```python
from build123d import *

# Parameters (mm, degrees)
F1_DEPTH   = 25.4
F2_DEPTH   = 6.35
F4_DEPTH   = 25.4
F5_DEPTH   = 25.4
F2_FACE2_W = 0.635
F2_FACE2_H = 6.35
F2_FACE3_W = 10.16
F2_FACE3_H = 6.35
F7_DEPTH   = 25.4
F9_DEPTH   = 25.4


with BuildPart() as f1:
    # F0 (on Top) → F1 (new body)
    with BuildSketch(Plane.XY):
        with BuildLine():
            ThreePointArc((1.2208780752, -0.3497952621), (1.2576595635, -0.1766137657), (1.27, 0))
            ThreePointArc((1.27, 0), (1.0317462976, 0.7405400579), (0.4063786184, 1.2032275007))
            ThreePointArc((0.4063786184, 1.2032275007), (0.0082488661, 1.2699732108), (-0.3907143254, 1.2084048642))
            ThreePointArc((-0.3907143254, 1.2084048642), (-1.1197739724, 0.5991713033), (-1.2221285, -0.3454011139))
            ThreePointArc((-1.2221285, -0.3454011139), (-1.0969705534, -0.6399653154), (-0.9021458423, -0.8938863906))
            ThreePointArc((-0.9021458423, -0.8938863906), (-0.0022842997, -1.2699979457), (0.8989244127, -0.897125911))
            ThreePointArc((0.8989244127, -0.897125911), (1.0946612978, -0.643907325), (1.2208780752, -0.3497952621))
        make_face()
    extrude(amount=F1_DEPTH)

    # F0 (on Top) → F2 (join)
    with BuildSketch(Plane.XY):
        with BuildLine():
            ThreePointArc((-0.9021458423, -0.8938863906), (-1.0969705534, -0.6399653154), (-1.2221285, -0.3454011139))
            Line((-1.2221285, -0.3454011139), (-10.0618945001, -5.3538077531))
            Line((-10.0618945001, -5.3538077531), (-9.7419118424, -5.9022930298))
            Line((-9.7419118424, -5.9022930298), (-0.9021458423, -0.8938863906))
        make_face()
        with BuildLine():
            ThreePointArc((-0.3907143254, 1.2084048642), (0.0082488661, 1.2699732108), (0.4063786184, 1.2032275007))
            Line((0.4063786184, 1.2032275007), (0.32674037, 11.3629153773))
            Line((0.32674037, 11.3629153773), (-0.3082387074, 11.3680701034))
            Line((-0.3082387074, 11.3680701034), (-0.3907143254, 1.2084048642))
        make_face()
        with BuildLine():
            Line((9.9781684573, -5.5010538621), (1.2208780752, -0.3497952621))
            ThreePointArc((1.2208780752, -0.3497952621), (1.0946612978, -0.643907325), (0.8989244127, -0.897125911))
            Line((0.8989244127, -0.897125911), (9.6562147948, -6.0483845109))
            Line((9.6562147948, -6.0483845109), (9.9781684573, -5.5010538621))
        make_face()
    extrude(amount=F2_DEPTH)

    # F3 (on face) → F4 (cut)
    with BuildSketch(Plane(origin=(0.1609768312, 0.2736653244, 0), x_dir=(-0.8619380297, 0.5070136417, 0), z_dir=(0.5070136417, 0.8619380297, 0))):
        Polygon((-11.3896722124, 0), (-3.303936429, 0), (-1.2296722124, 6.35), (-11.3896722124, 6.35), align=None)
    extrude(amount=-F4_DEPTH, mode=Mode.SUBTRACT)

    # F3 (on face) → F5 (cut)
    with BuildSketch(Plane(origin=(0.1609768312, 0.2736653244, 0), x_dir=(-0.8619380297, 0.5070136417, 0), z_dir=(0.5070136417, 0.8619380297, 0))):
        Polygon((-1.2296722124, 0), (-1.2296722124, 1.4659563295), (-3.303936429, 0), align=None)
    extrude(amount=-F5_DEPTH, mode=Mode.SUBTRACT)

    # F6 (on face) + F2_face2 (on face) + F2_face3 (on face) → F7 (cut)
    with BuildSketch(Plane(origin=(0.4157847513, 0.0032591916, 0), x_dir=(-0.0078384103, 0.9999692792, 0), z_dir=(0.9999692792, 0.0078384103, 0))):
        Polygon((1.2000051743, 6.35), (3.2617810744, 0), (11.3600051743, 0), (11.3600051743, 6.35), align=None)
        Polygon((3.2617810744, 0), (1.2000051743, 1.46235188), (1.2000051743, 0), align=None)
    with BuildSketch(Plane(origin=(0.0092508313, 11.3654927404, 3.175), x_dir=(-0.9999670511, 0.0081176789, 0), z_dir=(0.0081176789, 0.9999670511, 0))):
        Rectangle(F2_FACE2_W, F2_FACE2_H)
    with BuildSketch(Plane(origin=(-0.3494765164, 6.2882374838, 3.175), x_dir=(-0.0081176789, -0.9999670511, 0), z_dir=(-0.9999670511, 0.0081176789, 0))):
        Rectangle(F2_FACE3_W, F2_FACE3_H)
    extrude(amount=-F7_DEPTH, dir=(0.9999692792, 0.0078384103, 0), mode=Mode.SUBTRACT)

    # F8 (on face) → F9 (cut)
    with BuildSketch(Plane(origin=(-0.1488394932, 0.2626995742, 0), x_dir=(-0.8700557087, -0.4929534094, 0), z_dir=(-0.4929534094, 0.8700557087, 0))):
        Polygon((1.2335865348, 6.35), (3.295362435, 0), (11.3935865348, 0), (11.3935865348, 6.35), align=None)
        Polygon((3.295362435, 0), (1.2335865348, 1.46235188), (1.2335865348, 0), align=None)
    extrude(amount=-F9_DEPTH, mode=Mode.SUBTRACT)


solid = f1.part
```
Geometry: final body of the model. Coordinates: model frame, mm. A direction names the side the tool comes from. Round coordinates to 2 decimals unless told otherwise and drop trailing zeros. Order: outer loops, then holes, each group sorted by start corner. A loop starts at its lowest first (then second) coordinate and runs counter-clockwise, first axis right, second up. Notation, with made-up numbers: (42, -27) -> (70, -27) arc R21 ccw to (70, -23) -> close; hole circle Ø10 at (-32, 15). An arc over 180 degrees is marked (long way). Use one line per item in the form item = value. Start each with the question number.
1. Line query: probe 1 along Y at (x, z) = (0, 13.25); probe 2 along Y at (x, z) = (-1, 11.25); probe 3 along X at (y, z) = (0.35, 20). Output: solid intervals per line, ascending.
2. Cut plane A-A (z = 18.5). Return the cut outline in (x, y).
3. Cut plane D-D (z = 4.75). Return the cut outline in (x, y).
4. Draft query along X for faces 1 (the face through (1.944, -1.138, 0.743)), 2 (the face through (-1.95, -1.12, 3.22)), 3 (the face through (1.788, -0.683, 2.455)). Return one class per face: pulls with the +X half, pulls with the -X half, needs draft (parallel to the pull), parting line crosses it, or undercut.
5. Pin query (flat end, axial travel): pin 1 Ø1.5 at (x, z) = (0, 15) entering from +Y; pin 2 Ø1 at (y, z) = (2.5, 5.5) entering from -X; pin 3 Ø2 at (y, z) = (1.5, 21) entering from -X. Return the tip coordinate at first contact, or that it passes through.
6. Cut plane B-B (y = 2.15). Return the cut outline in (x, z), then the cut area to 3 significant figures.
7. Reachability of faces 4 (the face through (0, 0, 25.4)), 5 (the face through (-1.62, -1.3, 2.42)) from +Z, -Z, +X, -X, +Y, -Y: full face, straight path, thin tool, end or side. Return the list, or none.
8. Cut plane C-C (x = 2). Return the cut outline in (y, z), then the cut area to 3 significant figures.
Solution:
q1.probe_1 = -1.27 to 1.27
q1.probe_2 = -0.78 to 0.78
q1.probe_3 = -1.22 to 1.22
q2.outline = circle Ø2.54 at (0, 0)
q3.outline = (-1.67, -0.6) -> (-1.36, -1.15) -> (-0.9, -0.89) arc R1.27 ccw to (0.9, -0.9) -> (1.35, -1.16) -> (1.67, -0.61) -> (1.22, -0.35) arc R1.27 ccw to (0.41, 1.2) -> (0.4, 1.72) -> (-0.39, 1.72) -> (-0.39, 1.21) arc R1.27 ccw to (-1.22, -0.35) -> close
q4.face_1 = undercut
q4.face_2 = pulls with the -X half
q4.face_3 = pulls with the +X half
q5.pin_1 = 1.27
q5.pin_2 = through
q5.pin_3 = -1.17
q6.outline = (-0.38, 0.79) -> (0.4, 0.79) -> (0.4, 3.43) -> (-0.38, 3.42) -> close
q6.area = 2.06 mm^2
q7.face_4 = +Z, +X, -X, +Y, -Y
q7.face_5 = +Z, -Z, -Y
q8.outline = (-1.54, 0.56) -> (-0.81, 0.83) -> (-0.81, 3.58) -> (-1.54, 2.44) -> close
q8.area = 1.71 mm^2
